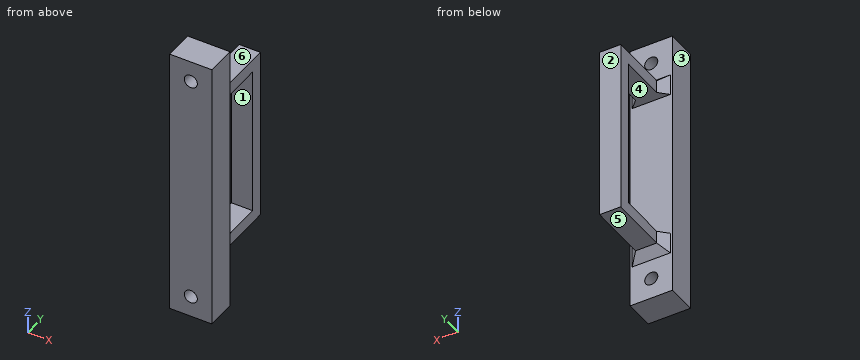
```python
from build123d import *

# Parameters (mm, degrees)
SKETCH1_W           = 10
SKETCH1_H           = 65
SKETCH1_R           = 1.55
BOSS_EXTRUDE1_DEPTH = 7
SKETCH2_W           = 5
SKETCH2_H           = 3
BOSS_EXTRUDE2_DEPTH = 16
SKETCH3_W           = 5
SKETCH3_H           = 3
BOSS_EXTRUDE3_DEPTH = 35.5
CHAMFER1_SIZE       = 2


with BuildPart() as part:
    # Sketch1 → Boss-Extrude1 (new body)
    with BuildSketch(Plane(origin=(0, 0, 0), x_dir=(1, 0, 0), z_dir=(0, 1, 0))):
        with Locations((5, 32.5)):
            Rectangle(SKETCH1_W, SKETCH1_H)
        with Locations((5, 60)):
            Circle(SKETCH1_R, mode=Mode.SUBTRACT)
        with Locations((5, 5)):
            Circle(SKETCH1_R, mode=Mode.SUBTRACT)
    extrude(amount=BOSS_EXTRUDE1_DEPTH)

    # Sketch2 → Boss-Extrude2 (add)
    with BuildSketch(Plane(origin=(0, 7, 0), x_dir=(1, 0, 0), z_dir=(0, 1, 0))):
        with Locations((5, 51.75)):
            Rectangle(SKETCH2_W, SKETCH2_H)
        with Locations((5, 13.25)):
            Rectangle(SKETCH2_W, SKETCH2_H)
    extrude(amount=BOSS_EXTRUDE2_DEPTH)

    # Sketch3 → Boss-Extrude3 (add)
    with BuildSketch(Plane.XY.offset(-50.25)):
        with Locations((5, 21.5)):
            Rectangle(SKETCH3_W, SKETCH3_H)
    extrude(amount=BOSS_EXTRUDE3_DEPTH)

    # Chamfer1
    chamfer1_edges = [part.edges().sort_by_distance(p)[0] for p in [
        (7.5, 7, -51.75),
        (5, 7, -53.25),
        (2.5, 7, -51.75),
        (7.5, 7, -13.25),
        (2.5, 7, -13.25),
        (5, 7, -11.75),
    ]]
    chamfer(chamfer1_edges, length=CHAMFER1_SIZE)


solid = part.part
```
Work out the finished part from the listing and answer in its coordinate system (mm). Face numbers are marked on the shaded views. A direction names the side the tool comes from. Coordinates: 2 decimals unless noted, no trailing zeros. Order: outer loops, then holes, each group sorted by start corner. A loop starts at its lowest first (then second) coordinate and runs counter-clockwise, first axis right, second up. Notation, with made-up numbers: M 78,89.5 L 90,89.5 A28 cw 90,120.5 Z; hole C 59,18 d3. An arc over 180 degrees is marked long. Use CSV: the item, a comma, the result in double quotes.
1) Section D-D on x = 1.5 is taken. Write down the section's boundary in (y, z), plus the area to 3 significant figures.
Worked out:
outline,"M 0,-65 L 7,-65 L 7,-55.25 L 8,-54.25 L 8,-50.25 L 7,-50.25 L 7,-14.75 L 8,-14.75 L 8,-10.75 L 7,-9.75 L 7,0 L 0,0 Z"
area,"464 mm^2"
2) Determine the mould class of the marked faces 1, 2 and 3 for opening direction Y: released by +Y, released by -Y, zero draft, split by the parting line, or undercut.
Worked out:
face 1,"undercut"
face 2,"released by +Y"
face 3,"zero draft"
3) Consider line 1 (Z direction, x = 5, y = 4.5); line 2 (X direction, y = 3.25, z = -5); line 3 (Y direction, x = 5.75, z = -20). Determine where each line is inside the solid, lowest interval first. Write a range as [from, to].
Worked out:
line 1,"z = [-65, -61.55], [-58.45, -6.55], [-3.45, 0]"
line 2,"x = [0, 3.45], [6.55, 10]"
line 3,"y = [0, 7], [20, 23]"
4) Section A-A on x = 5 is taken. Write down the section's boundary in (y, z).
Worked out:
outline,"M 0,-65 L 7,-65 L 7,-61.55 L 0,-61.55 Z; M 0,-58.45 L 7,-58.45 L 7,-55.25 L 9,-53.25 L 23,-53.25 L 23,-11.75 L 9,-11.75 L 7,-9.75 L 7,-6.55 L 0,-6.55 Z; M 0,-3.45 L 7,-3.45 L 7,0 L 0,0 Z; hole M 7,-50.25 L 20,-50.25 L 20,-14.75 L 7,-14.75 Z"
5) For the marked faces 4, 5 and 6, determine the directions among +Z, -Z, +X, -X, +Y, -Y from which every point of the face is accessible in a straight line to the end or side of a thin tool.
Worked out:
face 4,"+X, -X"
face 5,"-Z, +X, -X, +Y"
face 6,"+Z, +X, -X, +Y"
6) Section B-B on z = -5 is taken. Write down the section's boundary in (x, y), plus the area to 3 significant figures.
Worked out:
outline,"M 0,0 L 3.45,0 L 3.45,7 L 0,7 Z; M 6.55,0 L 10,0 L 10,7 L 6.55,7 Z"
area,"48.3 mm^2"
7) Section C-C on z = -54 is taken. Write down the section's boundary in (x, y), plus the area to 3 significant figures.
Worked out:
outline,"M 0,0 L 10,0 L 10,7 L 9.5,7 L 8.25,8.25 L 1.75,8.25 L 0.5,7 L 0,7 Z"
area,"79.7 mm^2"
8) Flat-ended cylindrical pins translate along their axes: pin 1 Ø2 at (x, y) = (5, 12.5) entering from +Z; pin 2 Ø5 at (x, z) = (5, -8) entering from +Y; pin 3 Ø6 at (y, z) = (17.5, -51.5) entering from +X. Find the tip coordinate at first contact, or state that the pin passes through.
Worked out:
pin 1,"stops at z = -11.75"
pin 2,"stops at y = 7.75"
pin 3,"stops at x = 7.5"
